Read the model definition and answer for the solid it produces. Units are mm, in the model's axes. Give positions to 0.01 mm unless a question says otherwise; leave off trailing zeros. Write each loop counter-clockwise with the first axis right and the second up, starting at its lowest first coordinate (ties: lowest second). Pieces come first, ordered by that corner, then holes. Notation, with made-up numbers: (63.5, 49.5) - (118.5, 49.5) arc R16 ccw to (118.5, 62.5) - close; hole circle Ø10 at (17.5, 25.25). An arc over 180 degrees is marked (long way). Answer as a JSON object with one key per item and string values. Group by question number.
Autodesk Inventor part; units mm, degrees
ref_plane "YZ Plane" through (0, 0, 0) normal (1, 0, 0) x (0, 1, 0)
ref_plane "XZ Plane" through (0, 0, 0) normal (0, 1, 0) x (-1, 0, 0)
ref_plane "XY Plane" through (0, 0, 0) normal (0, 0, 1) x (1, 0, 0)
sketch "Sketch1" plane through (0, 0, 0) normal (0, 0, 1) x (1, 0, 0)
  line L0 (0, 0) -> (31.75, 0)
  line L1 (31.75, 0) -> (31.75, -31.75)
  line L2 (31.75, -31.75) -> (0, -31.75)
  line L3 (0, -31.75) -> (0, 0)
  line L4 (28.575, -28.575) -> (28.575, -3.175)
  line L5 (28.575, -3.175) -> (3.175, -3.175)
  line L6 (3.175, -3.175) -> (3.175, -28.575)
  line L7 (3.175, -28.575) -> (28.575, -28.575)
  dimension "d0" = 31.75
  dimension "d1" = 3.175
extrude "Extrusion1" add sketch "Sketch1" along normal blind 1752.6
hole "Hole1" at (31.75, -15.875, 1733.55) direction (-1, 0, 0) diameter 6.731 end through all
hole "Hole2" at (31.75, -15.875, 19.05) direction (-1, 0, 0) diameter 6.731 end through all
properties part number "GE-12090-01"
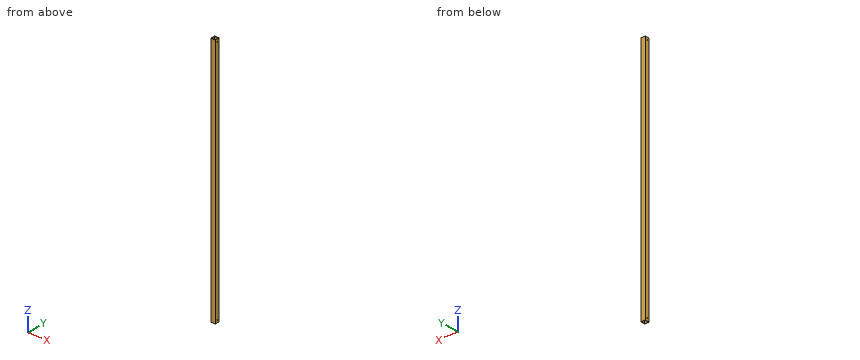
1) A flat-ended cylindrical pin translates along its axis: pin 1 Ø10 at (x, y) = (11, -21) entering from +Z. Find the tip coordinate at first contact, or state that the pin passes through.
2) Find the intervals of material crossed by line 1 (X direction, y = -14, z = 560.5) (3 decimals); line 2 (Y direction, x = 26, z = 1408) (3 decimals); line 3 (Y direction, x = 2, z = 19), in increasing order. Write a range as [from, to].
3) Find section B-B, the plane z = 710. Write down the section's boundary in (x, y) (3 decimals).
4) Find section A-A, the plane x = 10.5. Write down the section's boundary in (y, z) (3 decimals), and give its area (3 significant figures).
Values follow:
{
 "1": {"pin 1": "passes through"},
 "2": {"line 1": "x = [0, 3.175], [28.575, 31.75]", "line 2": "y = [-31.75, -28.575], [-3.175, 0]", "line 3": "y = [-31.75, -19.24], [-12.51, 0]"},
 "3": {"outline": "(0, -31.75) - (31.75, -31.75) - (31.75, 0) - (0, 0) - close; hole (3.175, -28.575) - (28.575, -28.575) - (28.575, -3.175) - (3.175, -3.175) - close"},
 "4": {"outline": "(-31.75, 0) - (-28.575, 0) - (-28.575, 1752.6) - (-31.75, 1752.6) - close; (-3.175, 0) - (0, 0) - (0, 1752.6) - (-3.175, 1752.6) - close", "area": "11,100 mm2"}
}
